Model file for the job. Use its own axes, mm. Face numbers are marked on the shaded views. Round coordinates to 2 decimals unless told otherwise and drop trailing zeros. Order: outer loops, then holes, each group sorted by start corner. A loop starts at its lowest first (then second) coordinate and runs counter-clockwise, first axis right, second up. Notation, with made-up numbers: (-22, -23.75) -> (9, -23.75) arc R18 ccw to (9, -0.75) -> close; hole circle Ø9 at (29.25, 80.25). An arc over 180 degrees is marked (long way). Put each result on its own line as item: value. Start each with the question number.
Q1. Cut at A-A, the plane z = 0. List the corners of the cut face in (x, y).
Q2. Probe L1, parallel to Z at x = -47.5, y = -11; L2, parallel to Y at x = 0, z = 73.25. List the from-to ranges inside material, lowest first.
Q3. Cut at D-D, the plane x = 47.5. List the corners of the cut face in (y, z).
Q4. Pull direction Z, two halves, no side cores. Call the marked faces 1, 2 and 3: released by +Z, released by -Z, zero draft, split by the parting line, or undercut.
Q5. Cut at C-C, the plane z = -47.5. List the corners of the cut face in (x, y), and give its area (3 significant figures).
Q6. Flat gauge pins, fed straight in: P1, Ø4, axis at y = -2, z = 60.5, coming from the +X side; P2, Ø3, axis at x = -47.5, z = -47.5, coming from the -Y side; P3, Ø2, axis at y = -4.5, z = 64.5, coming from the -X side; P4, Ø1, axis at x = 8, y = -3.5, coming from the -Z side. Where does each tip first touch, or does it go through?
Q7. Cut at B-B, the plane x = -32. List the corners of the cut face in (y, z).
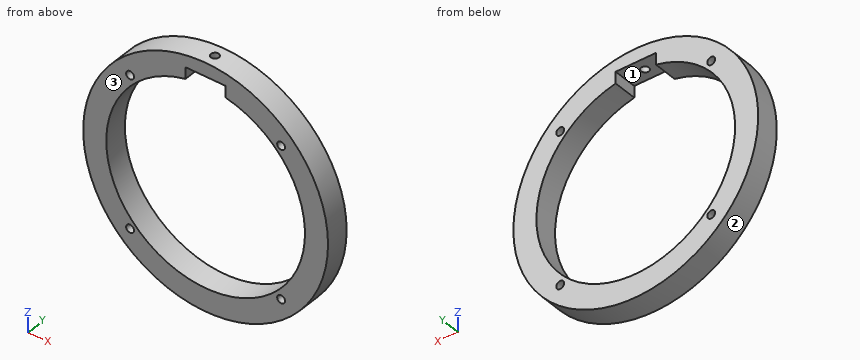
from build123d import *

# Parameters (mm, degrees)
F0_R     = 77
F0_R_2   = 62.5
F1_DEPTH = 15
F3_D     = 5
F5_DEPTH = 25
F7_D     = 5
F7_DEPTH = 12


with BuildPart() as f1:
    # F0 (on Front) → F1 (new body)
    with BuildSketch(Plane.XZ):
        Circle(F0_R)
        Circle(F0_R_2, mode=Mode.SUBTRACT)
    extrude(amount=F1_DEPTH)

    # F3 (through all)
    with Locations(Plane(origin=(0, 0, 0), x_dir=(1, 0, 0), z_dir=(0, 1, 0))):
        with Locations((-47.5, 47.5), (47.5, 47.5), (47.5, -47.5), (-47.5, -47.5)):
            Hole(F3_D / 2)

    # F4 (on face) → F5 (cut)
    with BuildSketch(Plane.XZ.offset(15)):
        with BuildLine():
            Line((12.658332, 68.463892), (-12.658332, 68.463892))
            Line((-12.658332, 68.463892), (-12.658332, 61.204711))
            ThreePointArc((-12.658332, 61.204711), (0, 62.5), (12.658332, 61.204711))
            Line((12.658332, 61.204711), (12.658332, 68.463892))
        make_face()
    extrude(amount=-F5_DEPTH, mode=Mode.SUBTRACT)

    # F7
    with Locations(Plane(origin=(0, 0, 68.463892), x_dir=(1, 0, 0), z_dir=(0, 0, -1))):
        with Locations((0, 7.5)):
            Hole(F7_D / 2, depth=F7_DEPTH)


solid = f1.part
Ans:
1. outline: (-77, -15) -> (-62.5, -15) -> (-62.5, 0) -> (-77, 0) -> close; (62.5, -15) -> (77, -15) -> (77, 0) -> (62.5, 0) -> close
2. L1: z = -60.6 to -50, -45 to -40.62, 40.62 to 45, 50 to 60.6
2. L2: y = -15 to -10, -5 to 0
3. outline: (-15, -60.6) -> (0, -60.6) -> (0, -50) -> (-15, -50) -> close; (-15, -45) -> (0, -45) -> (0, -40.62) -> (-15, -40.62) -> close; (-15, 40.62) -> (0, 40.62) -> (0, 45) -> (-15, 45) -> close; (-15, 50) -> (0, 50) -> (0, 60.6) -> (-15, 60.6) -> close
4. face 1: undercut
4. face 2: split by the parting line
4. face 3: zero draft
5. outline: (-60.6, -15) -> (-50, -15) -> (-50, 0) -> (-60.6, 0) -> close; (-45, -15) -> (-40.62, -15) -> (-40.62, 0) -> (-45, 0) -> close; (40.62, -15) -> (45, -15) -> (45, 0) -> (40.62, 0) -> close; (50, -15) -> (60.6, -15) -> (60.6, 0) -> (50, 0) -> close
5. area: 449 mm^2
6. P1: stops at x = 50.07
6. P2: passes through
6. P3: stops at x = -43.55
6. P4: stops at z = -76.63
7. outline: (-15, -70.04) -> (0, -70.04) -> (0, -53.69) -> (-15, -53.69) -> close; (-15, 53.69) -> (0, 53.69) -> (0, 70.04) -> (-15, 70.04) -> close
